```python
from build123d import *

# Parameters (mm, degrees)
F0_W     = 42
F0_H     = 85
F1_DEPTH = 3
F2_R     = 3
F4_DEPTH = 3
F5_R     = 1.5


with BuildPart() as f1:
    # F0 (on Front) → F1 (new body)
    with BuildSketch(Plane.XZ):
        with Locations((-12.290565, -9.565399)):
            Rectangle(F0_W, F0_H)
    extrude(amount=F1_DEPTH)

    # F2
    f2_edges = [f1.edges().sort_by_distance(p)[0] for p in [
        (-33.290565, -1.5, 32.934601),
        (8.709435, -1.5, 32.934601),
        (8.709435, -1.5, -52.065399),
        (-33.290565, -1.5, -52.065399),
    ]]
    fillet(f2_edges, radius=F2_R)

    # F3 (on face) → F4 (cut, through all)
    with BuildSketch(Plane(origin=(0, 0, 0), x_dir=(-1, 0, 0), z_dir=(0, 1, 0))):
        with BuildLine():
            Line((-5.459435, 8.759601), (-5.459435, 29.684601))
            Line((-5.459435, 29.684601), (3.540565, 29.684601))
            Line((3.540565, 29.684601), (3.540565, 32.934601))
            Line((3.540565, 32.934601), (-5.709435, 32.934601))
            ThreePointArc((-5.709435, 32.934601), (-7.830755, 32.055922), (-8.709435, 29.934601))
            Line((-8.709435, 29.934601), (-8.709435, 8.759601))
            Line((-8.709435, 8.759601), (-5.459435, 8.759601))
        make_face()
        with BuildLine():
            Line((21.040565, 32.934601), (21.040565, 29.684601))
            Line((21.040565, 29.684601), (30.040565, 29.684601))
            Line((30.040565, 29.684601), (30.040565, 8.759601))
            Line((30.040565, 8.759601), (33.290565, 8.759601))
            Line((33.290565, 8.759601), (33.290565, 29.934601))
            ThreePointArc((33.290565, 29.934601), (32.411885, 32.055922), (30.290565, 32.934601))
            Line((30.290565, 32.934601), (21.040565, 32.934601))
        make_face()
        with BuildLine():
            Line((33.290565, -27.890399), (30.040565, -27.890399))
            Line((30.040565, -27.890399), (30.040565, -48.815399))
            Line((30.040565, -48.815399), (21.040565, -48.815399))
            Line((21.040565, -48.815399), (21.040565, -52.065399))
            Line((21.040565, -52.065399), (30.290565, -52.065399))
            ThreePointArc((30.290565, -52.065399), (32.411885, -51.186719), (33.290565, -49.065399))
            Line((33.290565, -49.065399), (33.290565, -27.890399))
        make_face()
        with BuildLine():
            Line((-5.459435, -48.815399), (-5.459435, -27.890399))
            Line((-5.459435, -27.890399), (-8.709435, -27.890399))
            Line((-8.709435, -27.890399), (-8.709435, -49.065399))
            ThreePointArc((-8.709435, -49.065399), (-7.830755, -51.186719), (-5.709435, -52.065399))
            Line((-5.709435, -52.065399), (3.540565, -52.065399))
            Line((3.540565, -52.065399), (3.540565, -48.815399))
            Line((3.540565, -48.815399), (-5.459435, -48.815399))
        make_face()
    extrude(amount=-F4_DEPTH, mode=Mode.SUBTRACT)

    # F5
    f5_edges = [f1.edges().sort_by_distance(p)[0] for p in [
        (-12.290565, -3, 32.934601),
        (8.709435, -3, -9.565399),
        (-12.290565, -3, -52.065399),
        (-33.290565, -3, -9.565399),
    ]]
    fillet(f5_edges, radius=F5_R)


solid = f1.part
```
Source: CAD feature listing. Evaluate the final solid. Frame: model axes, mm. A direction names the side the tool comes from. Give positions to 0.01 mm unless a question says otherwise; leave off trailing zeros. Write each loop counter-clockwise with the first axis right and the second up, starting at its lowest first coordinate (ties: lowest second). Pieces come first, ordered by that corner, then holes. Notation, with made-up numbers: (23, 8) - (58, 8) arc R6 cw to (58, 12) - close; hole circle Ø7 at (13, 6.25). An arc over 180 degrees is marked (long way). One line per item, written item: value. Start each with the question number.
Q1. First-contact query: pin 1 Ø1.5 at (y, z) = (-1.5, -50.5) entering from -X; pin 2 Ø1.5 at (x, y) = (0, -1) entering from +Z; pin 3 Ø0.9 at (x, y) = (6.5, -1.5) entering from +Z. Flat tips, straight axial feed; report the tip coordinate or a pass-through.
Q2. Set-up query: faces 1 (the face through (1, -1, 29.685)), 2 (the face through (-32, -1, 8.76)), 3 (the face through (-30.041, -1, -38)), 4 (the face through (5.459, -1, -38)). Return all of +Z, -Z, +X, -X, +Y, -Y with unobstructed straight access to the full face (end or side cutting, diameter ignored); none if empty.
Q3. Material intervals for probe 1 along X at (y, z) = (-2.3, -43); probe 2 along Z at (x, y) = (-27, -1.6); probe 3 along Z at (x, y) = (-30.5, -0.25), sorted ascending. Write a range as from..to.
Q4. Section query C-C, the plane z = -33.5. Return the cut outline in (x, y).
Q5. Section query A-A, the plane y = -0.75. Return the cut outline in (x, z), then the cut area to 3 significant figures.
Q6. Section query B-B, the plane x = -22.5. Return the cut outline in (y, z).
Answer:
1. pin 1: stops at x = -21.04
1. pin 2: stops at z = 29.68
1. pin 3: stops at z = 8.76
2. face 1: +Z, +X, +Y, -Y
2. face 2: +Z, -X, +Y, -Y
2. face 3: -Z, -X, +Y, -Y
2. face 4: -Z, +X, +Y, -Y
3. probe 1: x = -30.04..5.46
3. probe 2: z = -48.82..29.68
3. probe 3: z = -27.89..8.76
4. outline: (-30.04, -3) - (5.46, -3) - (5.46, 0) - (-30.04, 0) - close
5. outline: (-33.29, -27.89) - (-30.04, -27.89) - (-30.04, -48.82) - (-21.04, -48.82) - (-21.04, -52.07) - (-3.54, -52.07) - (-3.54, -48.82) - (5.46, -48.82) - (5.46, -27.89) - (8.71, -27.89) - (8.71, 8.76) - (5.46, 8.76) - (5.46, 29.68) - (-3.54, 29.68) - (-3.54, 32.93) - (-21.04, 32.93) - (-21.04, 29.68) - (-30.04, 29.68) - (-30.04, 8.76) - (-33.29, 8.76) - close
5. area: 3,140 mm2
6. outline: (-3, -48.82) - (0, -48.82) - (0, 29.68) - (-3, 29.68) - close
